Can you work these out from the model? Positions are in its coordinate system, mm. A direction names the side the tool comes from. Give positions to 0.01 mm unless a question says otherwise; leave off trailing zeros. Write each loop counter-clockwise with the first axis right and the second up, starting at its lowest first coordinate (ties: lowest second). Pieces come first, ordered by that corner, then holes.
```python
from build123d import *

# Parameters (mm, degrees)
EXTRUDE_1_DEPTH     = 45
SKETCH_5_W          = 2
SKETCH_5_H          = 2
SKETCH_5_W_2        = 3
SKETCH_5_H_2        = 3
CUT_EXTRUDE_1_DEPTH = 4
SKETCH_6_R          = 0.6
CUT_EXTRUDE_2_DEPTH = 2
SKETCH_6_3_R        = 1
CUT_EXTRUDE_3_DEPTH = 1
CUT_EXTRUDE_START   = -48
SKETCH_6_4_R        = 0.6
CUT_EXTRUDE_4_DEPTH = 2
CUT_EXTRUDE_START_2 = -49
SKETCH_6_5_R        = 1
CUT_EXTRUDE_6_DEPTH = 1


with BuildPart() as part:
    # 草图4 → 凸台-拉伸1 (new body)
    with BuildSketch(Plane(origin=(0, 0, 0), x_dir=(1, 0, 0), z_dir=(0, 1, 0))):
        with BuildLine():
            Line((-25, 0), (-25, -3))
            Line((-25, -3), (25, -3))
            Line((25, -3), (25, 0))
            ThreePointArc((25, 0), (0, 8), (-25, 0))
        make_face()
    extrude(amount=EXTRUDE_1_DEPTH)

    # 草图5 → 切除-拉伸1 (cut)
    with BuildSketch(Plane.XY.offset(3)):
        with Locations((-22, 41.95)):
            Rectangle(SKETCH_5_W, SKETCH_5_H)
        with Locations((-19.5, 41.95)):
            Rectangle(SKETCH_5_W_2, SKETCH_5_H)
        with Locations((-22, 39.45)):
            Rectangle(SKETCH_5_W, SKETCH_5_H_2)
        with Locations((22, 41.95)):
            Rectangle(SKETCH_5_W, SKETCH_5_H)
        with Locations((19.5, 41.95)):
            Rectangle(SKETCH_5_W_2, SKETCH_5_H)
        with Locations((22, 39.45)):
            Rectangle(SKETCH_5_W, SKETCH_5_H_2)
        with Locations((-22, 3.05)):
            Rectangle(SKETCH_5_W, SKETCH_5_H)
        with Locations((-19.5, 3.05)):
            Rectangle(SKETCH_5_W_2, SKETCH_5_H)
        with Locations((-22, 5.55)):
            Rectangle(SKETCH_5_W, SKETCH_5_H_2)
        with Locations((22, 3.05)):
            Rectangle(SKETCH_5_W, SKETCH_5_H)
        with Locations((19.5, 3.05)):
            Rectangle(SKETCH_5_W_2, SKETCH_5_H)
        with Locations((22, 5.55)):
            Rectangle(SKETCH_5_W, SKETCH_5_H_2)
    extrude(amount=-CUT_EXTRUDE_1_DEPTH, mode=Mode.SUBTRACT)

    # 草图6 → 切除-拉伸2 (cut)
    with BuildSketch(Plane.ZY.offset(25)):
        with Locations((1.5, 5.55)):
            Circle(SKETCH_6_R)
        with Locations((1.5, 39.45)):
            Circle(SKETCH_6_R)
    extrude(amount=-CUT_EXTRUDE_2_DEPTH, mode=Mode.SUBTRACT)

    # 草图6<3> → 切除-拉伸3 (cut)
    with BuildSketch(Plane.ZY.offset(25)):
        with Locations((1.5, 5.55)):
            Circle(SKETCH_6_3_R)
        with Locations((1.5, 39.45)):
            Circle(SKETCH_6_3_R)
    extrude(amount=-CUT_EXTRUDE_3_DEPTH, mode=Mode.SUBTRACT)

    # 草图6<4> → 切除-拉伸4 (cut)
    with BuildSketch(Plane.ZY.offset(25).offset(CUT_EXTRUDE_START)):
        with Locations((1.5, 5.55)):
            Circle(SKETCH_6_4_R)
        with Locations((1.5, 39.45)):
            Circle(SKETCH_6_4_R)
    extrude(amount=-CUT_EXTRUDE_4_DEPTH, mode=Mode.SUBTRACT)

    # 草图6<5> → 切除-拉伸6 (cut)
    with BuildSketch(Plane.ZY.offset(25).offset(CUT_EXTRUDE_START_2)):
        with Locations((1.5, 5.55)):
            Circle(SKETCH_6_5_R)
        with Locations((1.5, 39.45)):
            Circle(SKETCH_6_5_R)
    extrude(amount=-CUT_EXTRUDE_6_DEPTH, mode=Mode.SUBTRACT)


solid = part.part
```
1) Please list where these lines run through material, in increasing order: L1, parallel to X at y = 4.5, z = 0.5; L2, parallel to Y at x = -22, z = -0.25; L3, parallel to Y at x = -23.15, z = 1.5.
Values follow:
L1: x = -25 to -23, -21 to 21, 23 to 25
L2: y = 0 to 2.05, 7.05 to 37.95, 42.95 to 45
L3: y = 0 to 4.95, 6.15 to 38.85, 40.05 to 45
2) If we mould it in two halves opening along Y, with no side actions, what happens to faces 5 (the face through (0, 0, -1)), 6 (the face through (-22, 7.05, 1)), 7 (the face through (25, 22, 2))? For each: +Y half, -Y half, draft (parallel to the pull), parting line (faces both ways), or undercut.
Values follow:
face 5: -Y half
face 6: undercut
face 7: draft
3) Suppose I cut it at C-C on x = 16. Write out the boundary of the cut face in (y, z).
Values follow:
outline: (0, -4.92) - (45, -4.92) - (45, 3) - (0, 3) - close
4) Suppose I cut it at B-B on y = 24. Write out the boundary of the cut face in (x, z) (1 decimal).
Values follow:
outline: (-25, 0) arc R43.1 ccw to (25, 0) - (25, 3) - (-25, 3) - close
5) For pin 1 Ø1 at (x, y) = (-17.5, 5.5) entering from -Z; pin 2 Ø0.7 at (y, z) = (5.55, 1.5) entering from -X; pin 3 Ø8 at (x, y) = (-3.5, 5) entering from -Z; pin 4 Ø1.9 at (y, z) = (39.45, 1.5) entering from +X, each with a flat end and sliding along its axis, tell me the tip position at first contact or that it passes through.
Values follow:
pin 1: stops at z = -4.5
pin 2: stops at x = -21
pin 3: stops at z = -8
pin 4: stops at x = 24
6) For faces 1 (the face through (0, 22, 3)), 2 (the face through (-23.507, 4.964, 1.37)), 3 (the face through (23.493, 38.864, 1.37)), 4 (the face through (18, 3, 1)), which set-ups out of +Z, -Z, +X, -X, +Y, -Y let a thin tool reach every point of the face, with its end or its side?
Values follow:
face 1: +Z, +X, -X, +Y, -Y
face 2: -X
face 3: +X
face 4: +Z
7) Suppose I cut it at A-A on y = 5.55. State how many separate pieces and enclosed holes the cut face has, plus the area to 3 significant figures.
Values follow:
separate pieces: 3
enclosed holes: 0
area: 400 mm2
